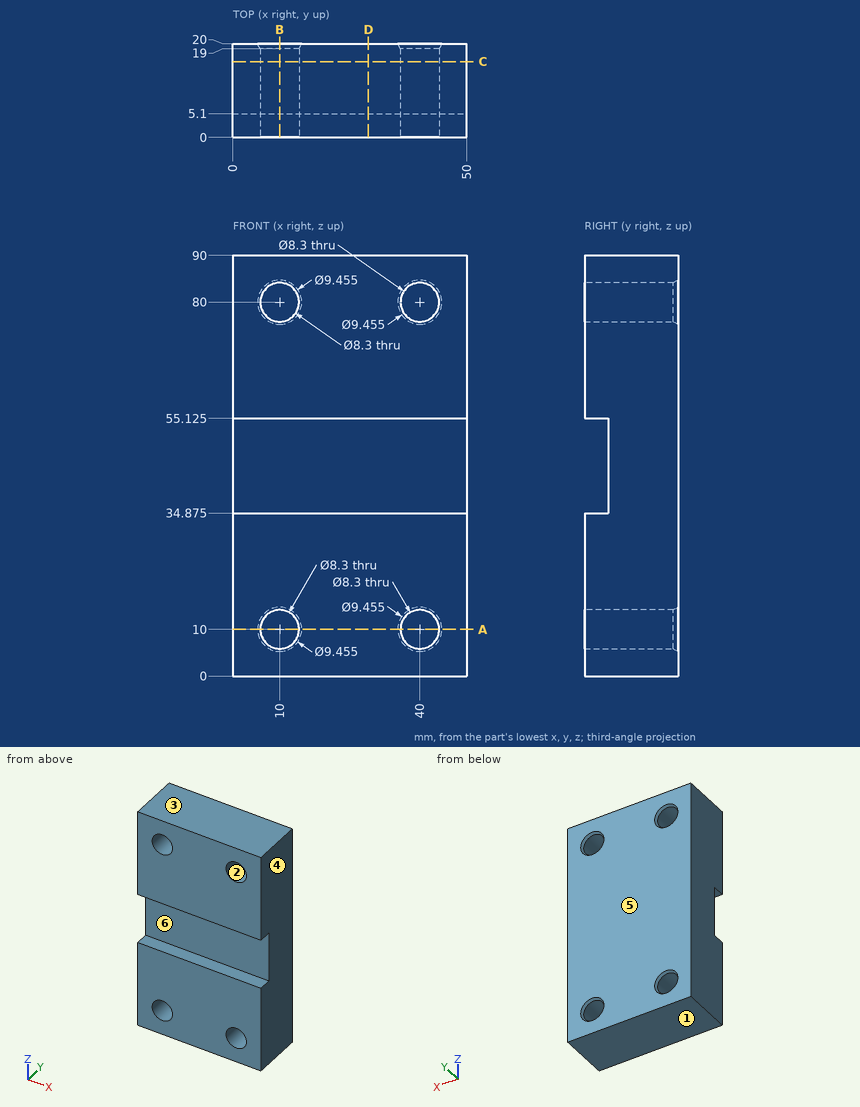
Part print with two shaded views. Sizes in mm from the minimum x, y, z corner. A direction names the side the tool comes from. Coordinates: 2 decimals unless noted, no trailing zeros. Write each loop counter-clockwise with the first axis right and the second up, starting at its lowest first coordinate (ties: lowest second). Pieces come first, ordered by that corner, then holes.
1. Band-saw the part on B-B, the plane x = 10. Give the number of separate pieces and of enclosed holes in the cut face, and give its area (3 significant figures).
Answer block:
separate pieces: 3
enclosed holes: 0
area: 1,360 mm2
2. Band-saw the part on D-D, the plane x = 29. Give the cut face in (y, z) (1 decimal), and give its area (3 significant figures).
Answer block:
outline: (0, 0) - (20, 0) - (20, 90) - (0, 90) - (0, 55.1) - (5.1, 55.1) - (5.1, 34.9) - (0, 34.9) - close
area: 1,700 mm2
3. Band-saw the part on C-C, the plane y = 16.25. Give the cut face in (x, z), and give its area (3 significant figures).
Answer block:
outline: (0, 0) - (50, 0) - (50, 90) - (0, 90) - close; hole circle Ø8.3 at (10, 10); hole circle Ø8.3 at (10, 80); hole circle Ø8.3 at (40, 10); hole circle Ø8.3 at (40, 80)
area: 4,280 mm2
4. Drop flat-ended pins along their axis: pin 1 (3 mm diameter, centred on y = 4, z = 64, fed in from -X); pin 2 (6.5 mm diameter, centred on x = 10, z = 10, fed in from +Y). Give the stop position or say it passes through.
Answer block:
pin 1: stops at x = 0
pin 2: passes through
5. Pull direction Z, two halves, no side cores. Call the marked faces 1, 2, 3 and 4: released by +Z, released by -Z, zero draft, split by the parting line, or undercut.
Answer block:
face 1: released by -Z
face 2: undercut
face 3: released by +Z
face 4: zero draft
6. Band-saw the part on A-A, the plane z = 10. Give the cut face in (x, y).
Answer block:
outline: (0, 0) - (5.85, 0) - (5.85, 19) - (5.27, 20) - (0, 20) - close; (14.15, 0) - (35.85, 0) - (35.85, 19) - (35.27, 20) - (14.73, 20) - (14.15, 19) - close; (44.15, 0) - (50, 0) - (50, 20) - (44.73, 20) - (44.15, 19) - close
7. Drill centre lines: probe 1 along X at (y, z) = (9.25, 10); probe 2 along Z at (x, y) = (2.5, 3.75) (1 decimal); probe 3 along Z at (x, y) = (43, 2.75) (1 decimal). Where is each one in solid material? Low to high.
Answer block:
probe 1: x = 0 to 5.85, 14.15 to 35.85, 44.15 to 50
probe 2: z = 0 to 34.9, 55.1 to 90
probe 3: z = 0 to 7.1, 12.9 to 34.9, 55.1 to 77.1, 82.9 to 90
8. 3-axis set-ups, long thin cutter, end or side, ignore diameter. For the marked faces 5 and 6: which of +Z, -Z, +X, -X, +Y, -Y reach the whole face in a straight line?
Answer block:
face 5: +Z, -Z, +X, -X, +Y
face 6: +X, -X, -Y
